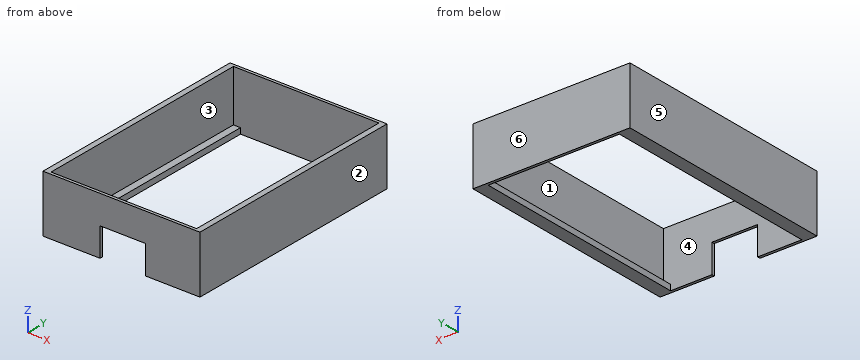
```python
from build123d import *

# Parameters (mm, degrees)
F1_DEPTH = 2
F2_DEPTH = 20
F0_W     = 16
F0_H     = 1
F3_DEPTH = 20
F4_DEPTH = 10


with BuildPart() as f1:
    # F0 (on Top) → F1 (new body)
    with BuildSketch(Plane.XY):
        Polygon((-23, -39), (-23, -35), (-23, 35), (-23, 39), (-25.5, 39), (-25.5, -39), align=None)
        Polygon((25.5, -39), (23, -39), (8.5, -39), (8.5, -40), (27.5, -40), (27.5, 40), (-27.5, 40), (-27.5, -40), (-7.5, -40), (-7.5, -39), (-23, -39), (-25.5, -39), (-25.5, 39), (-23, 39), (23, 39), (25.5, 39), align=None)
        Polygon((23, 35), (23, -35), (23, -39), (25.5, -39), (25.5, 39), (23, 39), align=None)
    extrude(amount=F1_DEPTH)

    # F0 (on Top) → F2 (join)
    with BuildSketch(Plane.XY):
        Polygon((25.5, -39), (23, -39), (8.5, -39), (8.5, -40), (27.5, -40), (27.5, 40), (-27.5, 40), (-27.5, -40), (-7.5, -40), (-7.5, -39), (-23, -39), (-25.5, -39), (-25.5, 39), (-23, 39), (23, 39), (25.5, 39), align=None)
    extrude(amount=F2_DEPTH)

    # F0 (on Top) → F3 (join)
    with BuildSketch(Plane.XY):
        with Locations((0.5, -39.5)):
            Rectangle(F0_W, F0_H)
    extrude(amount=F3_DEPTH)

    # F0 (on Top) → F4 (cut)
    with BuildSketch(Plane.XY):
        with Locations((0.5, -39.5)):
            Rectangle(F0_W, F0_H)
    extrude(amount=F4_DEPTH, mode=Mode.SUBTRACT)


solid = f1.part
```
Can you work these out from the model? Positions are in its coordinate system, mm. Face numbers are marked on the shaded views. A direction names the side the tool comes from. Give positions to 0.01 mm unless a question says otherwise; leave off trailing zeros. Order: outer loops, then holes, each group sorted by start corner. A loop starts at its lowest first (then second) coordinate and runs counter-clockwise, first axis right, second up. Notation, with made-up numbers: M 34.25,26.5 L 65.25,26.5 A6 cw 65.25,34.5 Z; hole C 15.5,-5.5 d3. An arc over 180 degrees is marked long. One line per item, written item: value.
1) I want a section at C-C, the plane z = 18.5. List the corners of the cut face in (x, y) for me, plus the area to 3 significant figures.
Answer sheet:
outline: M -27.5,-40 L 27.5,-40 L 27.5,40 L -27.5,40 Z; hole M -25.5,-39 L 25.5,-39 L 25.5,39 L -25.5,39 Z
area: 422 mm^2
2) I want a section at D-D, the plane z = 3.5. List the corners of the cut face in (x, y) for me.
Answer sheet:
outline: M -27.5,-40 L -7.5,-40 L -7.5,-39 L -25.5,-39 L -25.5,39 L 25.5,39 L 25.5,-39 L 8.5,-39 L 8.5,-40 L 27.5,-40 L 27.5,40 L -27.5,40 Z
3) On a 3-axis mill with a long thin cutter (end or side, diameter ignored), from which of +Z, -Z, +X, -X, +Y, -Y can I reach the whole of each face in a straight line? I mean the marked faces 1 and 2. Say none if no direction works.
Answer sheet:
face 1: +Z
face 2: +Z, -Z, +X, +Y, -Y
4) We'd pull the mould along X, two halves only. Please class the marked faces 3, 4, 5 and 6: released by +X, released by -X, zero draft, split by the parting line, or undercut.
Answer sheet:
face 3: undercut
face 4: undercut
face 5: released by -X
face 6: zero draft
5) For P1, Ø8, axis at x = 20, y = -8.5, coming from the +Z side; P2, Ø1.1, axis at x = 0.5, y = -39.5, coming from the -Z side, each with a flat end and sliding along its axis, tell me the tip position at first contact or that it passes through.
Answer sheet:
P1: stops at z = 2
P2: stops at z = 10
6) I want a section at A-A, the plane x = 6.5. List the corners of the cut face in (y, z) for me, plus the area to 3 significant figures.
Answer sheet:
outline: M -40,10 L -39,10 L -39,20 L -40,20 Z; M 39,0 L 40,0 L 40,20 L 39,20 Z
area: 30.0 mm^2
7) I want a section at B-B, the plane y = 21.5. List the corners of the cut face in (x, z) for me.
Answer sheet:
outline: M -27.5,0 L -23,0 L -23,2 L -25.5,2 L -25.5,20 L -27.5,20 Z; M 23,0 L 27.5,0 L 27.5,20 L 25.5,20 L 25.5,2 L 23,2 Z
8) Please list where these lines run through material, in increasing order: line 1 along X through (y, z) = (-8, 2.5); line 2 along Y through (x, z) = (-6, 13); line 3 along X through (y, z) = (-32.5, 1.25).
Answer sheet:
line 1: x = -27.5 to -25.5, 25.5 to 27.5
line 2: y = -40 to -39, 39 to 40
line 3: x = -27.5 to -23, 23 to 27.5
